from build123d import *

# Parameters (mm, degrees)
F0_W     = 80
F0_H     = 80
F1_DEPTH = 80
F2_R     = 4
F3_DEPTH = 5
F5_DEPTH = 2
F6_SIZE  = 5


with BuildPart() as f1:
    # F0 (on Top) → F1 (new body)
    with BuildSketch(Plane.XY):
        with Locations((-14.714826, 3.9e-05)):
            Rectangle(F0_W, F0_H)
    extrude(amount=F1_DEPTH)

    # F2 (on face) → F3 (join)
    with BuildSketch(Plane(origin=(0, 40.000039, 0), x_dir=(-1, 0, 0), z_dir=(0, 1, 0))):
        with Locations((0, 70)):
            Circle(F2_R)
        with Locations((-13.285174, 70)):
            Circle(F2_R)
    extrude(amount=F3_DEPTH)

    # F4 (on face) → F5 (cut)
    with BuildSketch(Plane(origin=(0, 40.000039, 0), x_dir=(-1, 0, 0), z_dir=(0, 1, 0))):
        with BuildLine():
            Line((39.714826, 50), (-10.285174, 50))
            Line((-10.285174, 50), (-10.285174, 30))
            ThreePointArc((-10.285174, 30), (-7.356242, 22.928932), (-0.285174, 20))
            Line((-0.285174, 20), (29.714826, 20))
            ThreePointArc((29.714826, 20), (36.785894, 22.928932), (39.714826, 30))
            Line((39.714826, 30), (39.714826, 50))
        make_face()
        with BuildLine():
            Line((-9.285174, 30), (-9.285174, 49))
            Line((-9.285174, 49), (38.714826, 49))
            Line((38.714826, 49), (38.714826, 30))
            ThreePointArc((38.714826, 30), (36.078787, 23.636039), (29.714826, 21))
            Line((29.714826, 21), (-0.285174, 21))
            ThreePointArc((-0.285174, 21), (-6.649135, 23.636039), (-9.285174, 30))
        make_face(mode=Mode.SUBTRACT)
    extrude(amount=-F5_DEPTH, mode=Mode.SUBTRACT)

    # F6
    f6_edges = [f1.edges().sort_by_distance(p)[0] for p in [
        (-14.714826, -39.999961, 0),
        (25.285174, 3.9e-05, 0),
        (25.285174, -39.999961, 40),
        (25.285174, 40.000039, 40),
        (25.285174, 3.9e-05, 80),
        (-54.714826, 40.000039, 40),
        (-14.714826, 40.000039, 0),
        (-54.714826, 3.9e-05, 0),
        (-54.714826, 3.9e-05, 80),
        (-14.714826, 40.000039, 80),
        (-14.714826, -39.999961, 80),
        (-54.714826, -39.999961, 40),
    ]]
    chamfer(f6_edges, length=F6_SIZE)


solid = f1.part
Model file for the job. Use its own axes, mm. A direction names the side the tool comes from. Coordinates: 2 decimals unless noted, no trailing zeros. Write each loop counter-clockwise with the first axis right and the second up, starting at its lowest first coordinate (ties: lowest second). Pieces come first, ordered by that corner, then holes. Notation, with made-up numbers: (4, 54.25) - (34, 54.25) arc R14 ccw to (34, 61.25) - close; hole circle Ø11 at (-31, -24.75). An arc over 180 degrees is marked (long way). Write each question's results on one line, items separated by ' | '. Start each with the question number.
1) 3-axis set-ups, long thin cutter, end or side, ignore diameter. For faces 1 (the face through (-36.15, 39.01, 23.71)), 2 (the face through (13, 45, 70)): which of +Z, -Z, +X, -X, +Y, -Y reach the whole face in a straight line?
2) Cut at A-A (z = 70). Write the cut outline in (x, y).
3) Cut at D-D (x = -48). Write the cut outline in (y, z), then the cut area to 3 significant figures.
4) Cut at C-C (z = 57). Write the cut outline in (x, y).
5) Mould opens along Z. For faces 3 (the face through (7.434, 39.014, 23.007)), 4 (the face through (-15, 40, 35)), 5 (the face through (0.867, 42.465, 66.095)) say: pulls with the +Z half, pulls with the -Z half, needs draft (parallel to the pull), parting line crosses it, or undercut.
6) Flat gauge pins, fed straight in: P1, Ø22.5, axis at x = -19.5, z = 39, coming from the +Y side; P2, Ø1, axis at y = 39.5, z = 42, coming from the -X side; P3, Ø1.6, axis at x = -17, y = 39.5, coming from the +Z side. Where does each tip first touch, or does it go through?
7) Probe line 1 along Y through (x, z) = (-3, 63); line 2 along Y through (x, z) = (-39, 42); line 3 along Z through (x, y) = (12.5, 39). List the from-to ranges inside material, lowest first. Write a range as from..to.
8) Cut at B-B (x = -25). Write the cut outline in (y, z), then the cut area to 3 significant figures.
Returned:
1) face 1: +Y | face 2: +Z, -Z, +X, -X, +Y
2) outline: (-54.71, -35) - (-49.71, -40) - (20.29, -40) - (25.29, -35) - (25.29, 35) - (20.29, 40) - (17.29, 40) - (17.29, 45) - (9.29, 45) - (9.29, 40) - (4, 40) - (4, 45) - (-4, 45) - (-4, 40) - (-49.71, 40) - (-54.71, 35) - close
3) outline: (-40, 5) - (-35, 0) - (35, 0) - (40, 5) - (40, 75) - (35, 80) - (-35, 80) - (-40, 75) - close | area: 6,350 mm^2
4) outline: (-54.71, -35) - (-49.71, -40) - (20.29, -40) - (25.29, -35) - (25.29, 35) - (20.29, 40) - (-49.71, 40) - (-54.71, 35) - close
5) face 3: undercut | face 4: needs draft | face 5: parting line crosses it
6) P1: y = 40 | P2: x = -50.71 | P3: z = 76.3
7) line 1: -40..40 | line 2: -40..38 | line 3: 4..76
8) outline: (-40, 5) - (-35, 0) - (35, 0) - (40, 5) - (40, 20) - (38, 20) - (38, 21) - (40, 21) - (40, 49) - (38, 49) - (38, 50) - (40, 50) - (40, 75) - (35, 80) - (-35, 80) - (-40, 75) - close | area: 6,350 mm^2
